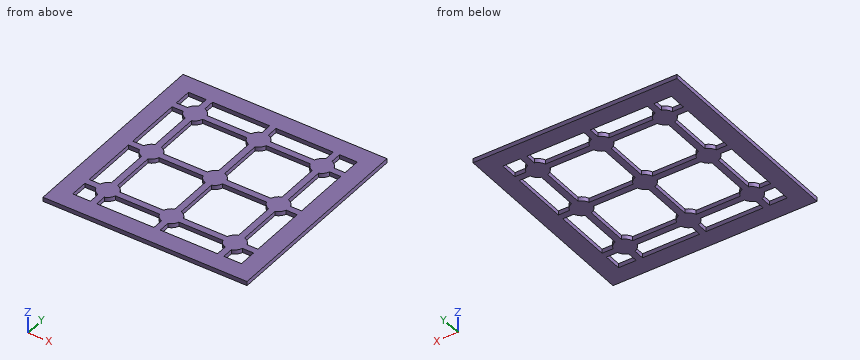
from build123d import *

# Parameters (mm, degrees)
BOSS_EXTRUDE2_DEPTH        = 0.12
CIRPATTERN2_COUNT          = 4
LPATTERN5_COUNT            = 2
LPATTERN5_PITCH            = 1.8
LPATTERN5_COPY_1_DEPTH     = 0.12
LPATTERN5_COPY_2_DEPTH     = 0.12
LPATTERN5_COPY_3_DEPTH     = 0.12
LPATTERN5_COL_COUNT        = 2
LPATTERN5_COL_PITCH        = 1.8
LPATTERN5_COL_COPY_1_DEPTH = 0.12
LPATTERN5_COL_COPY_2_DEPTH = 0.12
LPATTERN5_COL_COPY_3_DEPTH = 0.12
LPATTERN6_DEPTH            = 0.12
SKETCH3_W                  = 8
SKETCH3_H                  = 8
SKETCH3_W_2                = 4.78
SKETCH3_H_2                = 4.78
CUT_EXTRUDE8_DEPTH         = 4.820261771
SKETCH7_W                  = 5.78
SKETCH7_H                  = 5.78
SKETCH7_W_2                = 4.78
SKETCH7_H_2                = 4.78
BOSS_EXTRUDE3_DEPTH        = 0.12


# Read off the part's stored shape, not the designer's step: LPattern6
with BuildPart() as part:
    # Sketch2 → Boss-Extrude2 (new body)
    with BuildSketch(Plane.XY):
        with BuildLine():
            Line((0.09, 0.9), (0.09, 0.275680975))
            ThreePointArc((0.09, 0.275680975), (0, -0.29), (-0.09, 0.275680975))
            Line((-0.09, 0.275680975), (-0.09, 0.9))
            Line((-0.09, 0.9), (0.09, 0.9))
        make_face()
    boss_extrude2 = extrude(amount=BOSS_EXTRUDE2_DEPTH)

    # CirPattern2: Boss-Extrude2 ×4 about axis
    cirpattern2_axis = Axis((0, 0, 0), (0, 0, 1))
    for i in range(1, CIRPATTERN2_COUNT):
        add(boss_extrude2.rotate(cirpattern2_axis, i * 360 / CIRPATTERN2_COUNT))



with BuildPart() as lpattern5_1:
    # LPattern5: Boss-Extrude2 ×2
    with Locations(*[(0, i * LPATTERN5_PITCH, 0) for i in range(1, LPATTERN5_COUNT)]):
        add(boss_extrude2)

    # LPattern5 copy 1 sketch → LPattern5 copy 1 (add)
    with BuildSketch(Plane(origin=(0, 1.8, 0), x_dir=(0, 1, 0), z_dir=(0, 0, 1))):
        with BuildLine():
            Line((0.09, 0.9), (0.09, 0.275680975))
            ThreePointArc((0.09, 0.275680975), (0, -0.29), (-0.09, 0.275680975))
            Line((-0.09, 0.275680975), (-0.09, 0.9))
            Line((-0.09, 0.9), (0.09, 0.9))
        make_face()
    extrude(amount=LPATTERN5_COPY_1_DEPTH)


with BuildPart() as part_1:
    add(part.part)

    add(lpattern5_1.part)  # LPattern5 copy 2 merges LPattern5_1
    # LPattern5 copy 2 sketch → LPattern5 copy 2 (add)
    with BuildSketch(Plane(origin=(0, 1.8, 0), x_dir=(-1, 0, 0), z_dir=(0, 0, 1))):
        with BuildLine():
            Line((0.09, 0.9), (0.09, 0.275680975))
            ThreePointArc((0.09, 0.275680975), (0, -0.29), (-0.09, 0.275680975))
            Line((-0.09, 0.275680975), (-0.09, 0.9))
            Line((-0.09, 0.9), (0.09, 0.9))
        make_face()
    extrude(amount=LPATTERN5_COPY_2_DEPTH)

    # LPattern5 copy 3 sketch → LPattern5 copy 3 (add)
    with BuildSketch(Plane(origin=(0, 1.8, 0), x_dir=(0, -1, 0), z_dir=(0, 0, 1))):
        with BuildLine():
            Line((0.09, 0.9), (0.09, 0.275680975))
            ThreePointArc((0.09, 0.275680975), (0, -0.29), (-0.09, 0.275680975))
            Line((-0.09, 0.275680975), (-0.09, 0.9))
            Line((-0.09, 0.9), (0.09, 0.9))
        make_face()
    extrude(amount=LPATTERN5_COPY_3_DEPTH)

    # LPattern5 col: Boss-Extrude2 ×2
    with Locations(*[(0, -i * LPATTERN5_COL_PITCH, 0) for i in range(1, LPATTERN5_COL_COUNT)]):
        add(boss_extrude2)

    # LPattern5 col copy 1 sketch → LPattern5 col copy 1 (add)
    with BuildSketch(Plane(origin=(0, -1.8, 0), x_dir=(0, 1, 0), z_dir=(0, 0, 1))):
        with BuildLine():
            Line((0.09, 0.9), (0.09, 0.275680975))
            ThreePointArc((0.09, 0.275680975), (0, -0.29), (-0.09, 0.275680975))
            Line((-0.09, 0.275680975), (-0.09, 0.9))
            Line((-0.09, 0.9), (0.09, 0.9))
        make_face()
    extrude(amount=LPATTERN5_COL_COPY_1_DEPTH)

    # LPattern5 col copy 2 sketch → LPattern5 col copy 2 (add)
    with BuildSketch(Plane(origin=(0, -1.8, 0), x_dir=(-1, 0, 0), z_dir=(0, 0, 1))):
        with BuildLine():
            Line((0.09, 0.9), (0.09, 0.275680975))
            ThreePointArc((0.09, 0.275680975), (0, -0.29), (-0.09, 0.275680975))
            Line((-0.09, 0.275680975), (-0.09, 0.9))
            Line((-0.09, 0.9), (0.09, 0.9))
        make_face()
    extrude(amount=LPATTERN5_COL_COPY_2_DEPTH)

    # LPattern5 col copy 3 sketch → LPattern5 col copy 3 (add)
    with BuildSketch(Plane(origin=(0, -1.8, 0), x_dir=(0, -1, 0), z_dir=(0, 0, 1))):
        with BuildLine():
            Line((0.09, 0.9), (0.09, 0.275680975))
            ThreePointArc((0.09, 0.275680975), (0, -0.29), (-0.09, 0.275680975))
            Line((-0.09, 0.275680975), (-0.09, 0.9))
            Line((-0.09, 0.9), (0.09, 0.9))
        make_face()
    extrude(amount=LPATTERN5_COL_COPY_3_DEPTH)

    # LPattern6 outline → LPattern6 (add)
    with BuildSketch(Plane.XY):
        with BuildLine():
            Line((1.524319025, 0.09), (0.9, 0.09))
            Line((0.9, 0.09), (0.9, -0.09))
            Line((0.9, -0.09), (1.524319025, -0.09))
            ThreePointArc((1.524319025, -0.09), (1.594939033, -0.205060967), (1.71, -0.275680975))
            Line((1.71, -0.275680975), (1.71, -1.524319025))
            ThreePointArc((1.71, -1.524319025), (1.594939033, -1.594939033), (1.524319025, -1.71))
            Line((1.524319025, -1.71), (0.9, -1.71))
            Line((0.9, -1.71), (0.9, -1.89))
            Line((0.9, -1.89), (1.524319025, -1.89))
            ThreePointArc((1.524319025, -1.89), (1.594939033, -2.005060967), (1.71, -2.075680975))
            Line((1.71, -2.075680975), (1.71, -2.7))
            Line((1.71, -2.7), (1.89, -2.7))
            Line((1.89, -2.7), (1.89, -2.075680975))
            ThreePointArc((1.89, -2.075680975), (2.005060967, -2.005060967), (2.075680975, -1.89))
            Line((2.075680975, -1.89), (2.7, -1.89))
            Line((2.7, -1.89), (2.7, -1.71))
            Line((2.7, -1.71), (2.075680975, -1.71))
            ThreePointArc((2.075680975, -1.71), (2.005060967, -1.594939033), (1.89, -1.524319025))
            Line((1.89, -1.524319025), (1.89, -0.275680975))
            ThreePointArc((1.89, -0.275680975), (2.005060967, -0.205060967), (2.075680975, -0.09))
            Line((2.075680975, -0.09), (2.7, -0.09))
            Line((2.7, -0.09), (2.7, 0.09))
            Line((2.7, 0.09), (2.075680975, 0.09))
            ThreePointArc((2.075680975, 0.09), (2.005060967, 0.205060967), (1.89, 0.275680975))
            Line((1.89, 0.275680975), (1.89, 1.524319025))
            ThreePointArc((1.89, 1.524319025), (2.005060967, 1.594939033), (2.075680975, 1.71))
            Line((2.075680975, 1.71), (2.7, 1.71))
            Line((2.7, 1.71), (2.7, 1.89))
            Line((2.7, 1.89), (2.075680975, 1.89))
            ThreePointArc((2.075680975, 1.89), (2.005060967, 2.005060967), (1.89, 2.075680975))
            Line((1.89, 2.075680975), (1.89, 2.7))
            Line((1.89, 2.7), (1.71, 2.7))
            Line((1.71, 2.7), (1.71, 2.075680975))
            ThreePointArc((1.71, 2.075680975), (1.594939033, 2.005060967), (1.524319025, 1.89))
            Line((1.524319025, 1.89), (0.9, 1.89))
            Line((0.9, 1.89), (0.9, 1.71))
            Line((0.9, 1.71), (1.524319025, 1.71))
            ThreePointArc((1.524319025, 1.71), (1.594939033, 1.594939033), (1.71, 1.524319025))
            Line((1.71, 1.524319025), (1.71, 0.275680975))
            ThreePointArc((1.71, 0.275680975), (1.594939033, 0.205060967), (1.524319025, 0.09))
        make_face()
        with BuildLine():
            Line((-0.9, -0.09), (-0.9, 0.09))
            Line((-0.9, 0.09), (-1.524319025, 0.09))
            ThreePointArc((-1.524319025, 0.09), (-1.594939033, 0.205060967), (-1.71, 0.275680975))
            Line((-1.71, 0.275680975), (-1.71, 1.524319025))
            ThreePointArc((-1.71, 1.524319025), (-1.594939033, 1.594939033), (-1.524319025, 1.71))
            Line((-1.524319025, 1.71), (-0.9, 1.71))
            Line((-0.9, 1.71), (-0.9, 1.89))
            Line((-0.9, 1.89), (-1.524319025, 1.89))
            ThreePointArc((-1.524319025, 1.89), (-1.594939033, 2.005060967), (-1.71, 2.075680975))
            Line((-1.71, 2.075680975), (-1.71, 2.7))
            Line((-1.71, 2.7), (-1.89, 2.7))
            Line((-1.89, 2.7), (-1.89, 2.075680975))
            ThreePointArc((-1.89, 2.075680975), (-2.005060967, 2.005060967), (-2.075680975, 1.89))
            Line((-2.075680975, 1.89), (-2.7, 1.89))
            Line((-2.7, 1.89), (-2.7, 1.71))
            Line((-2.7, 1.71), (-2.075680975, 1.71))
            ThreePointArc((-2.075680975, 1.71), (-2.005060967, 1.594939033), (-1.89, 1.524319025))
            Line((-1.89, 1.524319025), (-1.89, 0.275680975))
            ThreePointArc((-1.89, 0.275680975), (-2.005060967, 0.205060967), (-2.075680975, 0.09))
            Line((-2.075680975, 0.09), (-2.7, 0.09))
            Line((-2.7, 0.09), (-2.7, -0.09))
            Line((-2.7, -0.09), (-2.075680975, -0.09))
            ThreePointArc((-2.075680975, -0.09), (-2.005060967, -0.205060967), (-1.89, -0.275680975))
            Line((-1.89, -0.275680975), (-1.89, -1.524319025))
            ThreePointArc((-1.89, -1.524319025), (-2.005060967, -1.594939033), (-2.075680975, -1.71))
            Line((-2.075680975, -1.71), (-2.7, -1.71))
            Line((-2.7, -1.71), (-2.7, -1.89))
            Line((-2.7, -1.89), (-2.075680975, -1.89))
            ThreePointArc((-2.075680975, -1.89), (-2.005060967, -2.005060967), (-1.89, -2.075680975))
            Line((-1.89, -2.075680975), (-1.89, -2.7))
            Line((-1.89, -2.7), (-1.71, -2.7))
            Line((-1.71, -2.7), (-1.71, -2.075680975))
            ThreePointArc((-1.71, -2.075680975), (-1.594939033, -2.005060967), (-1.524319025, -1.89))
            Line((-1.524319025, -1.89), (-0.9, -1.89))
            Line((-0.9, -1.89), (-0.9, -1.71))
            Line((-0.9, -1.71), (-1.524319025, -1.71))
            ThreePointArc((-1.524319025, -1.71), (-1.594939033, -1.594939033), (-1.71, -1.524319025))
            Line((-1.71, -1.524319025), (-1.71, -0.275680975))
            ThreePointArc((-1.71, -0.275680975), (-1.594939033, -0.205060967), (-1.524319025, -0.09))
            Line((-1.524319025, -0.09), (-0.9, -0.09))
        make_face()
    extrude(amount=LPATTERN6_DEPTH)

    # Sketch3 → Cut-Extrude8 (cut, through all)
    with BuildSketch(Plane.XY):
        Rectangle(SKETCH3_W, SKETCH3_H)
        Rectangle(SKETCH3_W_2, SKETCH3_H_2, mode=Mode.SUBTRACT)
    extrude(amount=CUT_EXTRUDE8_DEPTH, mode=Mode.SUBTRACT)

    # Sketch7 → Boss-Extrude3 (add)
    with BuildSketch(Plane.XY.offset(0.12)):
        Rectangle(SKETCH7_W, SKETCH7_H)
        Rectangle(SKETCH7_W_2, SKETCH7_H_2, mode=Mode.SUBTRACT)
    extrude(amount=-BOSS_EXTRUDE3_DEPTH)


solid = part_1.part
Design review of the part built by this model. Coordinates are the model's own, in mm. Round coordinates to 2 decimals unless told otherwise and drop trailing zeros. Write each loop counter-clockwise with the first axis right and the second up, starting at its lowest first coordinate (ties: lowest second). Pieces come first, ordered by that corner, then holes.
Item 1: Consider section A-A on y = 0.2. Give the boundary of the cut face in (x, z), and give its area (3 significant figures).
Item 2: Consider section C-C on z = 0.05. Count the separate pieces of the cut face and the enclosed holes in it, and give its area (3 significant figures).
Item 3: Wall thickness on L1, parallel to X at y = -0.8, z = 0.05: over which ranges is the line inside the solid? List them lowest first.
Item 4: For pin 1 Ø2 at (x, y) = (-1, 1) entering from -Z, flat-tipped, find the tip position at first contact; note if it passes through.
Check values:
1. outline: (-2.89, 0) - (-2.39, 0) - (-2.39, 0.12) - (-2.89, 0.12) - close; (-2.01, 0) - (-1.59, 0) - (-1.59, 0.12) - (-2.01, 0.12) - close; (-0.21, 0) - (0.21, 0) - (0.21, 0.12) - (-0.21, 0.12) - close; (1.59, 0) - (2.01, 0) - (2.01, 0.12) - (1.59, 0.12) - close; (2.39, 0) - (2.89, 0) - (2.89, 0.12) - (2.39, 0.12) - close
1. area: 0.271 mm2
2. separate pieces: 1
2. enclosed holes: 16
2. area: 16.3 mm2
3. L1: x = -2.89 to -2.39, -1.89 to -1.71, -0.09 to 0.09, 1.71 to 1.89, 2.39 to 2.89
4. pin 1: stops at z = 0
